Can you work these out from the model? Positions are in its coordinate system, mm. Face numbers are marked on the shaded views. A direction names the side the tool comes from. Give positions to 0.01 mm unless a question says otherwise; leave off trailing zeros. Order: outer loops, then holes, each group sorted by start corner. A loop starts at its lowest first (then second) coordinate and runs counter-clockwise, first axis right, second up. Notation, with made-up numbers: (41, -35.75) - (89, -35.75) arc R8 ccw to (89, -25.75) - close; hole circle Ø5 at (15.5, -6). An arc over 180 degrees is marked (long way). Use one line per item in the form item = value. Start each with the question number.
1) Which directions (+Z, -Z, +X, -X, +Y, -Y) give clear straight access to the entire face, cutting with the end or side of a thin tool? Please do the marked faces 1 and 2.
2) Please list where these lines run through material, in increasing order: probe 1 along X at (y, z) = (0, 123.2); probe 2 along X at (y, z) = (0, 119); probe 3 along Z at (x, y) = (-20, -12).
3) Suppose I cut it at C-C, the plane y = 23.5. Write out the boundary of the cut face in (x, z).
4) Suppose I cut it at B-B, the plane x = -44. Write out the boundary of the cut face in (y, z).
5) Suppose I cut it at D-D, the plane y = 44.5. Write out the boundary of the cut face in (x, z).
6) Suppose I cut it at A-A, the plane z = 84. Write out the boundary of the cut face in (x, y).
7) For pin 1 (3 mm diameter, centred on x = 32.5, y = 0.5, fed in from +Z); pin 2 (3 mm diameter, centred on x = -34, z = 93, fed in from +Y); pin 3 (4.5 mm diameter, centred on x = -44, y = 0, fed in from -Z), each with a flat end and sliding along its axis, tell me the tip position at first contact or that it passes through.
```python
from build123d import *

# Parameters (mm, degrees)
SKETCH265_R     = 60
PAD106_DEPTH    = 3
SKETCH266_R     = 3
SKETCH266_R_2   = 2
POCKET129_DEPTH = 3
SKETCH267_R     = 1.5
POCKET130_DEPTH = 13.001
PAD111_DEPTH    = 73.4


with BuildPart() as part:
    # Sketch005 → Revolution (revolve)
    with BuildSketch(Plane.XZ):
        with BuildLine():
            add(Edge.make_bspline(
                [(0, 112), (-7.388889, 112), (-19, 122)],
                knots=[0, 0, 0, 1.023749, 1.023749, 1.023749], degree=2, weights=[1, 1.133893, 1]))
            Line((-19, 122), (0, 122))
            Line((0, 122), (0, 112))
        make_face()
    revolve(axis=Axis((0, 0, 0), (0, 0, 1)))

    # Sketch265 (on Face2 of Revolution) → Pad106 (new body)
    with BuildSketch(Plane(origin=(0, 0, 122), x_dir=(-1, 0, 0), z_dir=(0, 0, 1))):
        Circle(SKETCH265_R)
    extrude(amount=PAD106_DEPTH)

    # Sketch266 (on Face3 of Pad106) → Pocket129 (cut)
    with BuildSketch(Plane(origin=(0, 0, 125), x_dir=(-1, 0, 0), z_dir=(0, 0, 1))):
        Circle(SKETCH266_R)
        with Locations((-32, 0)):
            Circle(SKETCH266_R)
        with Locations((32, 0)):
            Circle(SKETCH266_R)
        with Locations((-44, 0)):
            Circle(SKETCH266_R_2)
        with Locations((44, 0)):
            Circle(SKETCH266_R_2)
    extrude(amount=-POCKET129_DEPTH, mode=Mode.SUBTRACT)

    # Sketch267 (on Face3 of Pocket129) → Pocket130 (cut, through all)
    with BuildSketch(Plane(origin=(0, 0, 125), x_dir=(-1, 0, 0), z_dir=(0, 0, 1))):
        Circle(SKETCH267_R)
    extrude(amount=-POCKET130_DEPTH, mode=Mode.SUBTRACT)

    # Sketch274 (on Face2 of Pocket130) → Pad111 (join)
    with BuildSketch(Plane(origin=(0, 0, 122), x_dir=(1, 0, 0), z_dir=(0, 0, -1))):
        Polygon((-29.10452, -0.958487), (-29.722186, 2.028316), (-32.617666, 2.986802), (-34.89548, 0.958487), (-34.277814, -2.028316), (-31.382334, -2.986802), align=None)
        Polygon((34.433148, -1.839101), (34.809282, 1.187617), (32.376134, 3.026718), (29.566852, 1.839101), (29.190718, -1.187617), (31.623866, -3.026718), align=None)
    extrude(amount=PAD111_DEPTH)


with BuildPart() as part_1:
    # Body001 placement: moved
    add(part.part.moved(Location((0, 0, -0.6))))


solid = part_1.part
```
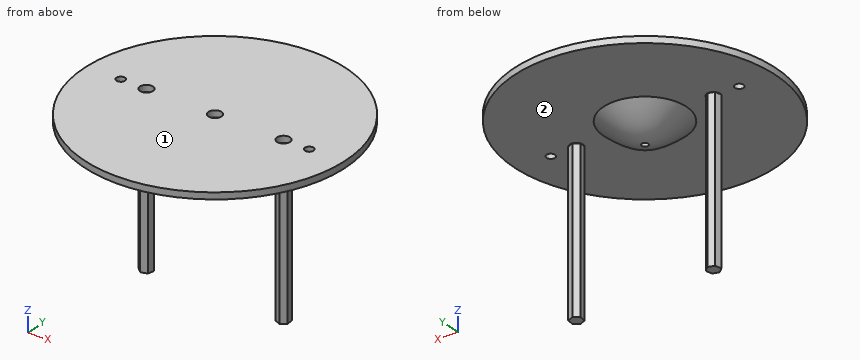
Result sheet:
q1.face_1 = +Z, +X, -X, +Y, -Y
q1.face_2 = -Z
q2.probe_1 = -60 to -46, -42 to -35, -29 to -3, 3 to 29, 35 to 42, 46 to 60
q2.probe_2 = -34.7 to -29.3, -16.12 to -1.5, 1.5 to 16.12, 29.34 to 34.66
q2.probe_3 = 121.4 to 124.4
q3.outline = (-55.21, 121.4) - (55.21, 121.4) - (55.21, 124.4) - (-55.21, 124.4) - close
q4.outline = (-40.79, 121.4) - (-2, 121.4) - (-2, 124.4) - (-40.79, 124.4) - close; (2, 121.4) - (40.79, 121.4) - (40.79, 124.4) - (2, 124.4) - close
q5.outline = (-40.25, 121.4) - (40.25, 121.4) - (40.25, 124.4) - (-40.25, 124.4) - close
q6.outline = (-34.9, -0.96) - (-32.62, -2.99) - (-29.72, -2.03) - (-29.1, 0.96) - (-31.38, 2.99) - (-34.28, 2.03) - close; (29.19, 1.19) - (29.57, -1.84) - (32.38, -3.03) - (34.81, -1.19) - (34.43, 1.84) - (31.62, 3.03) - close
q7.pin_1 = 121.4
q7.pin_2 = 2.62
q7.pin_3 = 121.4
